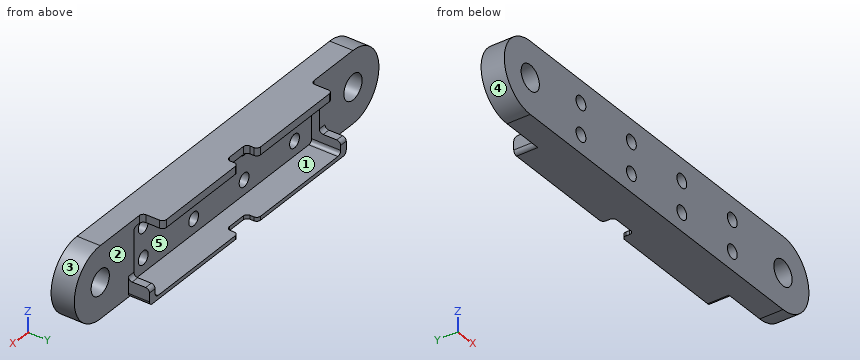
```python
from build123d import *

# Parameters (mm, degrees)
SKETCH1_W           = 35.1
SKETCH1_H           = 18.5
BOSS_EXTRUDE1_DEPTH = 11.5
SKETCH7_W           = 33.1
SKETCH7_H           = 15.5
CUT_EXTRUDE5_DEPTH  = 7.5
SKETCH2_R           = 1.75
CUT_EXTRUDE1_DEPTH  = 39.076534769
SKETCH4_W           = 14.25
SKETCH4_H           = 5.5
CUT_EXTRUDE3_DEPTH  = 5
SKETCH8_R           = 3.25
BOLT_EXTRUDE_DEPTH  = 6
FILLET3_R           = 1
SKETCH9_W           = 7
SKETCH9_H           = 18.5
CUT_EXTRUDE6_DEPTH  = 3
FILLET6_R           = 1


with BuildPart() as part:
    # Sketch1 → Boss-Extrude1 (new body)
    with BuildSketch(Plane(origin=(0, 0, 0), x_dir=(1, 0, 0), z_dir=(0, 1, 0))):
        with Locations((-17.55, 0)):
            Rectangle(SKETCH1_W, SKETCH1_H)
    extrude(amount=BOSS_EXTRUDE1_DEPTH)

    # Sketch7 → Cut-Extrude5 (cut)
    with BuildSketch(Plane(origin=(0, 11.5, 0), x_dir=(1, 0, 0), z_dir=(0, 1, 0))):
        with Locations((-16.55, 0.5)):
            Rectangle(SKETCH7_W, SKETCH7_H)
    extrude(amount=-CUT_EXTRUDE5_DEPTH, mode=Mode.SUBTRACT)

    # Sketch2 → Cut-Extrude1 (cut, through all)
    with BuildSketch(Plane(origin=(0, 0, 0), x_dir=(-1, 0, 0), z_dir=(0, 1, 0))):
        with Locations(Location((27, 3.5, 0), (0, 0, 270))):
            Circle(SKETCH2_R)
        with Locations(Location((9, 3.5, 0), (0, 0, 270))):
            Circle(SKETCH2_R)
        with Locations(Location((27, -4.5, 0), (0, 0, 270))):
            Circle(SKETCH2_R)
        with Locations(Location((9, -4.5, 0), (0, 0, 270))):
            Circle(SKETCH2_R)
    extrude(amount=CUT_EXTRUDE1_DEPTH, mode=Mode.SUBTRACT)

    # Sketch4 → Cut-Extrude3 (cut)
    with BuildSketch(Plane.ZY.offset(35.1)):
        with Locations((2.125, 8.75)):
            Rectangle(SKETCH4_W, SKETCH4_H)
    extrude(amount=-CUT_EXTRUDE3_DEPTH, mode=Mode.SUBTRACT)

    # Sketch8 → bolt extrude (add)
    with BuildSketch(Plane(origin=(0, 0, 0), x_dir=(-1, 0, 0), z_dir=(0, -1, 0))):
        with BuildLine():
            Line((35.1, -9.25), (45.1, -9.25))
            ThreePointArc((45.1, -9.25), (54.35, 0), (45.1, 9.25))
            Line((45.1, 9.25), (35.1, 9.25))
            Line((35.1, 9.25), (35.1, -9.25))
        make_face()
        with Locations(Location((45.1, 0, 0), (0, 0, 90))):
            Circle(SKETCH8_R, mode=Mode.SUBTRACT)
    extrude(amount=-BOLT_EXTRUDE_DEPTH)

    # Mirror1: part across plane


with BuildPart() as part_1:
    add(part.part)
    add(part.part.mirror(Plane(origin=(0, 0, 0), x_dir=(0, 0, 1), z_dir=(1, 0, 0))))

    # Fillet3
    fillet3_edges = [part_1.edges().sort_by_distance(p)[0] for p in [
        (-34.1, 6, -5),
        (-34.1, 11.5, -5),
        (-30.1, 11.5, 8.25),
        (-30.1, 6, 8.25),
        (34.1, 11.5, -5),
        (34.1, 6, -5),
        (30.1, 11.5, 8.25),
        (30.1, 6, 8.25),
    ]]
    fillet(fillet3_edges, radius=FILLET3_R)

    # Sketch9 → Cut-Extrude6 (cut)
    with BuildSketch(Plane(origin=(0, 11.5, 0), x_dir=(1, 0, 0), z_dir=(0, 1, 0))):
        Rectangle(SKETCH9_W, SKETCH9_H)
    extrude(amount=-CUT_EXTRUDE6_DEPTH, mode=Mode.SUBTRACT)

    # Fillet6
    fillet6_edges = [part_1.edges().sort_by_distance(p)[0] for p in [
        (-33.1, 7.75, -8.25),
        (-33.1, 5, 7.25),
        (-3.5, 8.5, -8.75),
        (-3.5, 8.5, 8.25),
        (3.5, 8.5, -8.75),
        (3.5, 8.5, 8.25),
        (-3.5, 11.5, -8.75),
        (3.5, 11.5, -8.75),
        (3.5, 11.5, 8.25),
        (-3.5, 11.5, 8.25),
        (-35.1, 8.75, -9.25),
        (35.1, 8.75, -9.25),
        (33.1, 7.75, -8.25),
        (33.1, 5, 7.25),
    ]]
    fillet(fillet6_edges, radius=FILLET6_R)


solid = part_1.part
```
The listing builds one solid part. Answer for the finished solid, in the listing's coordinates (mm). Face numbers are marked on the shaded views. A direction names the side the tool comes from. Coordinates: 2 decimals unless noted, no trailing zeros. Loops run counter-clockwise (first coordinate to the right, second up) from the corner with the lowest first, then second, coordinate; pieces in that order, holes last. Notation, with made-up numbers: M 50,65.5 L 90,65.5 A29 cw 90,85.5 Z; hole C 1,82.25 d1. An arc over 180 degrees is marked long. Answer as CSV lines item,"result". Start each with the question number.
(1) Find the intervals of material crossed by L1, parallel to Z at x = 9, y = 1.6; L2, parallel to X at y = 1.8, z = 0; L3, parallel to X at y = 3, z = -4.5, in increasing order. Write a range as [from, to].
(2) The mould has two halves that part along X. Classify the marked faces 1, 2 and 3: pulls with the +X half, pulls with the -X half, needs draft (parallel to the pull), parting line crosses it, or undercut.
(3) The part is cut by section C-C (y = 2.75). State how many separate pieces and enclosed holes the cut face has, and give its area (3 significant figures).
(4) The part is cut by section D-D (x = 19). Give the vertices of the cut face in (y, z), and give its area (3 significant figures).
(5) The part is cut by section B-B (x = -27). Give the vertices of the cut face in (y, z), and give its area (3 significant figures).
(6) For the marked faces 4 and 5, determine the directions among +Z, -Z, +X, -X, +Y, -Y from which every point of the face is accessible in a straight line to the end or side of a thin tool.
(7) Given pin 1 (4.5 mm diameter, centred on x = 7, z = -1.5, fed in from +Y); pin 2 (0.8 mm diameter, centred on y = 10, z = -9, fed in from -X); pin 3 (1 mm diameter, centred on x = -0.5, z = 8.5, fed in from +Y), each flat-ended and moving along its own axis, determine where each tip first touches the part or whether it passes through.
(8) The part is cut by section A-A (z = 0). Give the vertices of the cut face in (x, y), and give its area (3 significant figures).
Determined:
1,L1,"[-9.25, -6.25], [-2.75, 1.75], [5.25, 9.25]"
1,L2,"[-54.35, -48.35], [-41.85, 41.85], [48.35, 54.35]"
1,L3,"[-53.18, -28.75], [-25.25, -10.75], [-7.25, 7.25], [10.75, 25.25], [28.75, 53.18]"
2,face 1,"undercut"
2,face 2,"needs draft"
2,face 3,"pulls with the +X half"
3,separate pieces,"1"
3,enclosed holes,"10"
3,area,"1,790 mm2"
4,outline,"M 0,-9.25 L 11.5,-9.25 L 11.5,-8.25 L 4,-8.25 L 4,7.25 L 11.5,7.25 L 11.5,9.25 L 0,9.25 Z"
4,area,"96.5 mm2"
5,outline,"M 0,-9.25 L 11.5,-9.25 L 11.5,-8.25 L 4,-8.25 L 4,-6.25 L 0,-6.25 Z; M 0,-2.75 L 4,-2.75 L 4,1.75 L 0,1.75 Z; M 0,5.25 L 4,5.25 L 4,7.25 L 11.5,7.25 L 11.5,9.25 L 0,9.25 Z"
5,area,"68.5 mm2"
6,face 4,"-X, +Y, -Y"
6,face 5,"+Y"
7,pin 1,"y = 4"
7,pin 2,"x = -35.04"
7,pin 3,"y = 8.5"
8,outline,"M -54.35,0 L -48.35,0 L -48.35,6 L -54.35,6 Z; M -41.85,0 L 41.85,0 L 41.85,6 L 33.1,6 L 33.1,4 L -33.1,4 L -33.1,6 L -41.85,6 Z; M 48.35,0 L 54.35,0 L 54.35,6 L 48.35,6 Z"
8,area,"442 mm2"
